Check sheet for the drawn part. Datum: minimum x, y, z corner. Units: mm. A direction names the side the tool comes from. Coordinates: 2 decimals unless noted, no trailing zeros. Order: outer loops, then holes, each group sorted by start corner. A loop starts at its lowest first (then second) coordinate and runs counter-clockwise, first axis right, second up. Notation, with made-up numbers: (-31.75, -12.75) - (-1.75, -12.75) arc R37 ccw to (-1.75, 25.25) - close; hole circle Ø9 at (-10, -30.5). An arc over 180 degrees is marked (long way). One line per item, written item: value. Start each with the question number.
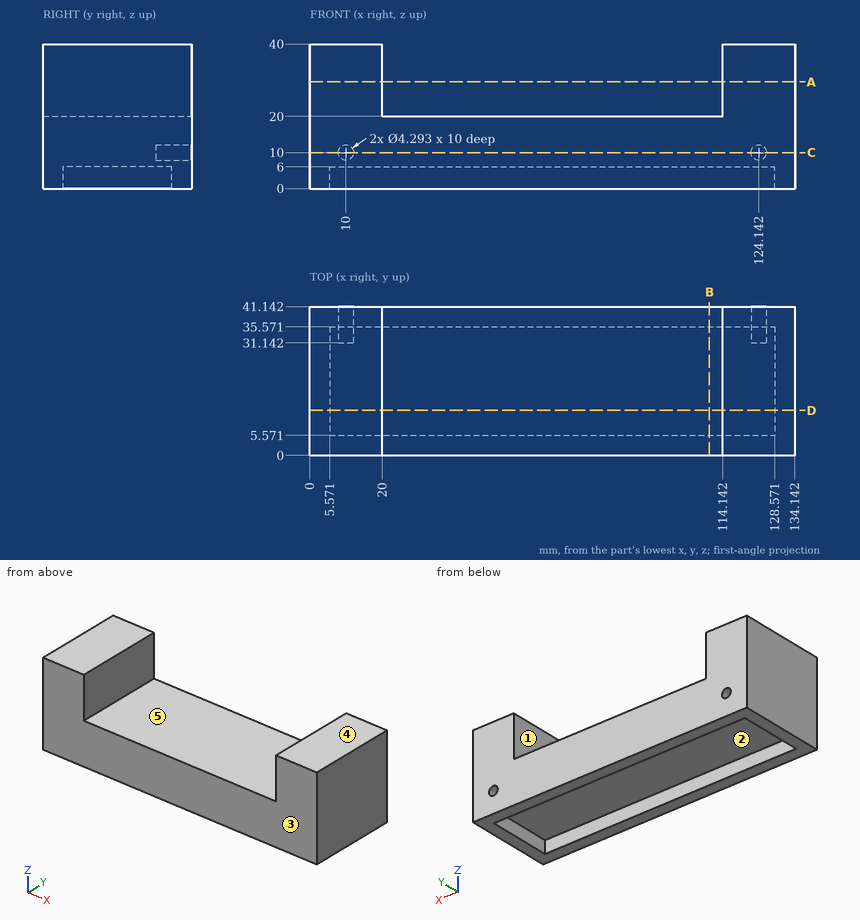
Q1. Cross-section at A-A, the plane z = 29.5. Enter the section's corners in (x, y).
Q2. Cross-section at D-D, the plane y = 12.5. Enter the section's corners in (x, z), and give its area (4 significant figures).
Q3. Cross-section at B-B, the plane x = 110.5. Enter the section's corners in (y, z), and give its area (3 significant figures).
Q4. Release check for a two-part mould opening along Y. For the marked faces 1, 2 and 3 record: released by +Y, released by -Y, zero draft, split by the parting line, or undercut.
Q5. Set-up check for the marked faces 4 and 5: record each of +Z, -Z, +X, -X, +Y, -Y from which the full face is reachable in a straight line by a thin tool's end or side.
Q6. Cross-section at C-C, the plane z = 10. Enter the section's corners in (x, y), and give its area (3 significant figures).
Q7. Material ranges on probe 1 along Z at (x, y) = (10, 38); probe 2 along Y at (x, z) = (18, 5); probe 3 along X at (y, z) = (37.5, 23.5), recorded low to high.
Q8. Gauge pin test, flat ends, axial feed: P1, Ø20.5, axis at x = 55, y = 30, coming from the +Z side; P2, Ø1.3, axis at x = 10, z = 11, coming from the +Y side. Record the tip position at first contact, or that the pin passes through.
Check result:
1. outline: (0, 0) - (20, 0) - (20, 41.14) - (0, 41.14) - close; (114.14, 0) - (134.14, 0) - (134.14, 41.14) - (114.14, 41.14) - close
2. outline: (0, 0) - (5.57, 0) - (5.57, 6) - (128.57, 6) - (128.57, 0) - (134.14, 0) - (134.14, 40) - (114.14, 40) - (114.14, 20) - (20, 20) - (20, 40) - (0, 40) - close
2. area: 2,745 mm2
3. outline: (0, 0) - (5.57, 0) - (5.57, 6) - (35.57, 6) - (35.57, 0) - (41.14, 0) - (41.14, 20) - (0, 20) - close
3. area: 643 mm2
4. face 1: zero draft
4. face 2: undercut
4. face 3: released by -Y
5. face 4: +Z, +X, -X, +Y, -Y
5. face 5: +Z, +Y, -Y
6. outline: (0, 0) - (134.14, 0) - (134.14, 41.14) - (126.29, 41.14) - (126.29, 31.14) - (122, 31.14) - (122, 41.14) - (12.15, 41.14) - (12.15, 31.14) - (7.85, 31.14) - (7.85, 41.14) - (0, 41.14) - close
6. area: 5,430 mm2
7. probe 1: z = 0 to 7.85, 12.15 to 40
7. probe 2: y = 0 to 5.57, 35.57 to 41.14
7. probe 3: x = 0 to 20, 114.14 to 134.14
8. P1: stops at z = 20
8. P2: stops at y = 31.14
